```python
from build123d import *

# Parameters (mm, degrees)
SKETCH1_W           = 5
SKETCH1_H           = 60
BOSS_EXTRUDE1_DEPTH = 5
BOSS_EXTRUDE2_START = 5
SKETCH1_3_R         = 5
SKETCH1_3_W         = 5
SKETCH1_3_H         = 60
BOSS_EXTRUDE2_DEPTH = 5
BOSS_EXTRUDE3_START = -5
SKETCH1_4_R         = 5
SKETCH1_4_W         = 5
SKETCH1_4_H         = 60
BOSS_EXTRUDE3_DEPTH = 5
BOSS_EXTRUDE4_DEPTH = 10
FILLET3_R           = 5
FILLET2_R           = 2
SKETCH4_R           = 7.5
CUT_EXTRUDE1_DEPTH  = 15


with BuildPart() as part:
    # Sketch1 → Boss-Extrude1 (new body, symmetric)
    with BuildSketch(Plane.XY):
        with Locations((-13, 0)):
            Rectangle(SKETCH1_W, SKETCH1_H)
    extrude(amount=BOSS_EXTRUDE1_DEPTH, both=True)

    # Sketch1<3> → Boss-Extrude2 (add)
    with BuildSketch(Plane.XY.offset(BOSS_EXTRUDE2_START)):
        with BuildLine():
            Line((0, 30), (-10.5, 30))
            Line((-10.5, 30), (-10.5, -30))
            Line((-10.5, -30), (0, -30))
            ThreePointArc((0, -30), (7.071067812, -27.071067812), (10, -20))
            Line((10, -20), (10, 20))
            ThreePointArc((10, 20), (7.071067812, 27.071067812), (0, 30))
        make_face()
        with Locations((0, -20)):
            Circle(SKETCH1_3_R, mode=Mode.SUBTRACT)
        with Locations((0, 20)):
            Circle(SKETCH1_3_R, mode=Mode.SUBTRACT)
        with Locations((-13, 0)):
            Rectangle(SKETCH1_3_W, SKETCH1_3_H)
    extrude(amount=BOSS_EXTRUDE2_DEPTH)

    # Sketch1<4> → Boss-Extrude3 (add)
    with BuildSketch(Plane.XY.offset(BOSS_EXTRUDE3_START)):
        with BuildLine():
            Line((0, 30), (-10.5, 30))
            Line((-10.5, 30), (-10.5, -30))
            Line((-10.5, -30), (0, -30))
            ThreePointArc((0, -30), (7.071067812, -27.071067812), (10, -20))
            Line((10, -20), (10, 20))
            ThreePointArc((10, 20), (7.071067812, 27.071067812), (0, 30))
        make_face()
        with Locations((0, -20)):
            Circle(SKETCH1_4_R, mode=Mode.SUBTRACT)
        with Locations((0, 20)):
            Circle(SKETCH1_4_R, mode=Mode.SUBTRACT)
        with Locations((-13, 0)):
            Rectangle(SKETCH1_4_W, SKETCH1_4_H)
    extrude(amount=-BOSS_EXTRUDE3_DEPTH)

    # Sketch3 → Boss-Extrude4 (add, symmetric)
    with BuildSketch(Plane(origin=(0, 0, 0), x_dir=(1, 0, 0), z_dir=(0, 1, 0))):
        with BuildLine():
            Line((-15.5, -10), (-15.5, 10))
            ThreePointArc((-15.5, 10), (-23.153668647, 8.47759065), (-29.642135624, 4.142135624))
            Line((-29.642135624, 4.142135624), (-43.784271247, -10))
            Line((-43.784271247, -10), (-29.642135624, -24.142135624))
            Line((-29.642135624, -24.142135624), (-15.5, -10))
        make_face()
    extrude(amount=BOSS_EXTRUDE4_DEPTH, both=True)

    # Fillet3
    fillet3_edges = [part.edges().sort_by_distance(p)[0] for p in [
        (-22.571067812, -10, 17.071067812),
        (-23.153668647, -10, -8.47759065),
        (-36.713203436, -10, 2.928932188),
        (-22.571067812, 10, 17.071067812),
        (-23.153668647, 10, -8.47759065),
        (-36.713203436, 10, 2.928932188),
    ]]
    fillet(fillet3_edges, radius=FILLET3_R)

    # Fillet2
    fillet2_edges = [part.edges().sort_by_distance(p)[0] for p in [
        (-15.5, 30, 0),
        (-15.5, -30, 0),
    ]]
    fillet(fillet2_edges, radius=FILLET2_R)

    # Sketch4 → Cut-Extrude1 (cut)
    with BuildSketch(Plane(origin=(-26.892135624, 0, 26.892135624), x_dir=(0.707106781, 0, 0.707106781), z_dir=(-0.707106781, 0, 0.707106781))):
        with Locations((-13.889087297, 0)):
            Circle(SKETCH4_R)
    extrude(amount=-CUT_EXTRUDE1_DEPTH, mode=Mode.SUBTRACT)


solid = part.part
```
Can you work these out from the model? Positions are in its coordinate system, mm. A direction names the side the tool comes from. Coordinates: 2 decimals unless noted, no trailing zeros. Loops run counter-clockwise (first coordinate to the right, second up) from the corner with the lowest first, then second, coordinate; pieces in that order, holes last.
1) Imagine slicing it at A-A on y = -22.5. List the corners of the cut face in (x, z) for me, plus the area to 3 significant figures.
2) For pin 1 (5 mm diameter, centred on y = 11, z = 1.5, fed in from +X); pin 2 (13 mm diameter, centred on x = -6, y = -1, fed in from +Z); pin 3 (4 mm diameter, centred on y = -13, z = 10, fed in from -X), each with a flat end and sliding along its axis, tell me the tip position at first contact or that it passes through.
3) Imagine slicing it at B-B on x = 2. List the corners of the cut face in (y, z) for me.
4) I need wall thicknesses on probe 1 along Y at (x, z) = (0, -8.5); probe 2 along Y at (x, z) = (-32, 12); probe 3 along Z at (x, y) = (3.5, -1.5). Which ranges of each line are inside material? Lowest first, please.
5) Thinking about a two-plate mould opening in Y: for faces 1 (the cylindrical face through (6.99, -27.15, 7.46)), 2 (the flat face through (-26.18, 0.11, 6.39)), 3 (the cylindrical face through (-23.707, 8.574, 16.081)), which applies, pulls with the +Y half, pulls with the -Y half, needs draft (parallel to the pull), parting line crosses it, or undercut?
6) Which directions (+Z, -Z, +X, -X, +Y, -Y) give clear straight access to the entire face, cutting with the end or side of a thin tool? Please do faces 4 (the cylindrical face through (-23.652, -8.496, 16.136)), 5 (the flat face through (-10.5, 0, 0)), 6 (the cylindrical face through (-1.08, 15.12, 7.46)), 7 (the flat face through (-28, 10, 8)).
Completed:
1. outline: (-15.5, -10) - (-4.33, -10) - (-4.33, -5) - (-10.5, -5) - (-10.5, 5) - (-4.33, 5) - (-4.33, 10) - (-15.5, 10) - close; (4.33, -10) - (9.68, -10) - (9.68, -5) - (4.33, -5) - close; (4.33, 5) - (9.68, 5) - (9.68, 10) - (4.33, 10) - close
1. area: 215 mm2
2. pin 1: stops at x = -10.5
2. pin 2: stops at z = 10
2. pin 3: stops at x = -15.5
3. outline: (-29.8, -10) - (-24.58, -10) - (-24.58, -5) - (-29.8, -5) - close; (-29.8, 5) - (-24.58, 5) - (-24.58, 10) - (-29.8, 10) - close; (-15.42, -10) - (15.42, -10) - (15.42, -5) - (-15.42, -5) - close; (-15.42, 5) - (15.42, 5) - (15.42, 10) - (-15.42, 10) - close; (24.58, -10) - (29.8, -10) - (29.8, -5) - (24.58, -5) - close; (24.58, 5) - (29.8, 5) - (29.8, 10) - (24.58, 10) - close
4. probe 1: y = -30 to -25, -15 to 15, 25 to 30
4. probe 2: y = -10 to -7.5, 7.5 to 10
4. probe 3: z = -10 to -5, 5 to 10
5. face 1: pulls with the -Y half
5. face 2: undercut
5. face 3: pulls with the +Y half
6. face 4: +Z, -Y
6. face 5: +X, +Y, -Y
6. face 6: +Z, -Z
6. face 7: +Z, -Z, -X, +Y
